```python
from build123d import *

# Parameters (mm, degrees)
SKETCH1_R           = 1.5
BOSS_EXTRUDE1_DEPTH = 3
SKETCH2_W           = 1.5
SKETCH2_H           = 3
BOSS_EXTRUDE2_DEPTH = 5
BOSS_EXTRUDE3_DEPTH = 3
BOSS_EXTRUDE4_START = -1.5
BOSS_EXTRUDE4_DEPTH = 5
SKETCH6_OUTSIDE_W   = 36.314
SKETCH6_OUTSIDE_H   = 49.814
CUT_EXTRUDE2_DEPTH  = 57.984647055
SKETCH7_R           = 1
CUT_EXTRUDE3_DEPTH  = 62.010245195


with BuildPart() as part:
    # Sketch1 → Boss-Extrude1 (new body)
    with BuildSketch(Plane(origin=(0, 0, 0), x_dir=(1, 0, 0), z_dir=(0, 1, 0))):
        with BuildLine():
            Line((-10, 0), (-10, 20))
            Line((-10, 20), (-5, 20))
            Line((-5, 20), (-5, 8.660254038))
            ThreePointArc((-5, 8.660254038), (8.660254038, -5), (-10, 0))
        make_face()
        with Locations(Location((0, 0, 0), (0, 0, 270))):
            Circle(SKETCH1_R, mode=Mode.SUBTRACT)
    extrude(amount=BOSS_EXTRUDE1_DEPTH)

    # Sketch2 → Boss-Extrude2 (add)
    with BuildSketch(Plane.ZY.offset(10)):
        with Locations((-19.25, 1.5)):
            Rectangle(SKETCH2_W, SKETCH2_H)
        Polygon((-18.5, 0), (-17, 0), (-6.5, 0), (-6.5, 3), (-18.5, 3), align=None)
        Polygon((-18.5, 30), (-18.5, 3), (-6.5, 3), (-17, 13.5), (-17, 30), align=None)
        Polygon((-20, 3), (-18.5, 3), (-18.5, 30), (-20, 30), (-30, 30), (-30, 27), (-30.5, 27), (-20, 16.5), align=None)
    extrude(amount=-BOSS_EXTRUDE2_DEPTH)

    # Sketch4 → Boss-Extrude3 (add)
    with BuildSketch(Plane(origin=(0, 30, 0), x_dir=(1, 0, 0), z_dir=(0, 1, 0))):
        with BuildLine():
            Line((-5, 17), (-10, 17))
            Line((-10, 17), (-10, 40))
            ThreePointArc((-10, 40), (-7.071067812, 47.071067812), (0, 50))
            Line((0, 50), (0, 35))
            Line((0, 35), (-5, 37.886751346))
            Line((-5, 37.886751346), (-5, 30))
            Line((-5, 30), (-5, 17))
        make_face()
    extrude(amount=-BOSS_EXTRUDE3_DEPTH)

    # Sketch5 → Boss-Extrude4 (add, symmetric)
    with BuildSketch(Plane(origin=(0, 30, 0), x_dir=(1, 0, 0), z_dir=(0, 1, 0)).offset(BOSS_EXTRUDE4_START)):
        with BuildLine():
            Line((-5, 37.886751346), (-10, 37.886751346))
            Line((-10, 37.886751346), (-10, 40))
            ThreePointArc((-10, 40), (-7.071067812, 47.071067812), (0, 50))
            Line((0, 50), (7.642881742, 50))
            Line((7.642881742, 50), (0, 35))
            Line((0, 35), (-5, 37.886751346))
        make_face()
    extrude(amount=BOSS_EXTRUDE4_DEPTH, both=True)

    # Sketch6 outside → Cut-Extrude2 (cut, through all)
    with BuildSketch(Plane.XY.offset(-35)):
        with Locations((0, 16.75)):
            Rectangle(SKETCH6_OUTSIDE_W, SKETCH6_OUTSIDE_H)
        with BuildLine():
            Line((-10, 30), (-5, 30))
            ThreePointArc((-5, 30), (1.559200766, 30.891151362), (7.642881742, 33.5))
            Line((7.642881742, 33.5), (7.642881742, 23.5))
            ThreePointArc((7.642881742, 23.5), (1.559200766, 26.108848638), (-5, 27))
            Line((-5, 27), (-10, 27))
            Line((-10, 27), (-10, 30))
        make_face(mode=Mode.SUBTRACT)
    extrude(amount=-CUT_EXTRUDE2_DEPTH, mode=Mode.SUBTRACT)

    # Sketch7 → Cut-Extrude3 (cut, through all)
    with BuildSketch(Plane.XZ):
        with Locations(Location((0, -7.5, 0), (0, 0, 270))):
            Circle(SKETCH7_R)
        with Locations(Location((0, 7.5, 0), (0, 0, 270))):
            Circle(SKETCH7_R)
    extrude(amount=-CUT_EXTRUDE3_DEPTH, mode=Mode.SUBTRACT)


solid = part.part
```
Input: part model. Units: mm. Frame: model coordinates. A direction names the side the tool comes from. Coordinates: 2 decimals unless noted, no trailing zeros. Loops run counter-clockwise (first coordinate to the right, second up) from the corner with the lowest first, then second, coordinate; pieces in that order, holes last. Notation, with made-up numbers: (38, -25) - (66, -25) arc R21 cw to (66, 4) - close; hole circle Ø3 at (49.5, 69). An arc over 180 degrees is marked (long way). Answer in a Markdown table with one row per item.
(1) Pin query (flat end, axial travel): P1, Ø6, axis at x = -1.5, y = 24.5, coming from the -Z side; P2, Ø1.6, axis at x = 0, z = -7.5, coming from the -Y side; P3, Ø3, axis at x = -4.5, y = 7, coming from the -Z side; P4, Ø6, axis at x = 1.5, z = -2, coming from the +Y side. Return the tip coordinate at first contact, or that it passes through.
Model answer:
| item | result |
|---|---|
| P1 | stops at z = -50 |
| P2 | passes through |
| P3 | stops at z = -20 |
| P4 | stops at y = 3 |
(2) Cut plane D-D on z = -18.5. Output: boundary loops of the cut face in (x, y).
Model answer:
| item | result |
|---|---|
| outline | (-10, 0) - (-5, 0) - (-5, 30) - (-10, 30) - close |
(3) Cut plane B-B on y = 25. Output: boundary loops of the cut face in (x, z), plus the area to 3 significant figures.
Model answer:
| item | result |
|---|---|
| outline | (-10, -28.5) - (-5, -28.5) - (-5, -17) - (-10, -17) - close; (4.71, -50) - (7.64, -50) - (4.71, -44.25) - close |
| area | 65.9 mm² |
(4) Mould query, pull axis X, two halves, no side actions, for faces 1 (the face through (-2, 0, -2)), 2 (the face through (-0.6, 1.5, -6.7)), 3 (the face through (4.724, 28.57, -44.272)). Classes: pulls with the +X half, pulls with the -X half, needs draft (parallel to the pull), parting line crosses it, or undercut.
Model answer:
| item | result |
|---|---|
| face 1 | needs draft |
| face 2 | undercut |
| face 3 | pulls with the +X half |
(5) Set-up query: faces 4 (the face through (-8, 30, -33)), 5 (the face through (-8, 22, -17)), 6 (the face through (-8, 8, -20)). Return all of +Z, -Z, +X, -X, +Y, -Y with unobstructed straight access to the full face (end or side cutting, diameter ignored); none if empty.
Model answer:
| item | result |
|---|---|
| face 4 | +Z, -Z, -X, +Y |
| face 5 | +Z, +X, -X, +Y |
| face 6 | -Z, +X, -X, -Y |
(6) Cut plane C-C on x = 5.5. Output: boundary loops of the cut face in (y, z), plus the area to 3 significant figures.
Model answer:
| item | result |
|---|---|
| outline | (0, -8.35) - (3, -8.35) - (3, 8.35) - (0, 8.35) - close; (24.64, -50) - (32.36, -50) - (32.36, -45.79) - (24.64, -45.79) - close |
| area | 82.5 mm² |
(7) Material intervals for L1, parallel to X at y = 0.8, z = -7.5; L2, parallel to X at y = 1, z = 7; L3, parallel to Y at x = -4.5, z = -42.5, sorted ascending. Write a range as from..to.
Model answer:
| item | result |
|---|---|
| L1 | x = -10..-1, 1..6.61 |
| L2 | x = -7.14..-0.87, 0.87..7.14 |
| L3 | y = 26.99..30.01 |
(8) Cut plane A-A on z = 7.5. Output: boundary loops of the cut face in (x, y), plus the area to 3 significant figures.
Model answer:
| item | result |
|---|---|
| outline | (-6.61, 0) - (-1, 0) - (-1, 3) - (-6.61, 3) - close; (1, 0) - (6.61, 0) - (6.61, 3) - (1, 3) - close |
| area | 33.7 mm² |
